Design review of the part built by this model. Coordinates are the model's own, in mm. A direction names the side the tool comes from. Give positions to 0.01 mm unless a question says otherwise; leave off trailing zeros. Order: outer loops, then holes, each group sorted by start corner. A loop starts at its lowest first (then second) coordinate and runs counter-clockwise, first axis right, second up. Notation, with made-up numbers: (11.5, -26) -> (43.5, -26) arc R35 cw to (43.5, 10) -> close; hole circle Ø4 at (33.5, 73.5). An arc over 180 degrees is marked (long way). Return JSON: item names as keys, results as strings.
```python
from build123d import *

# Parameters (mm, degrees)
F0_W     = 254
F0_H     = 100
F1_DEPTH = 25.4
F2_W     = 254
F2_H     = 100
F2_R     = 27.9579286296
F3_DEPTH = 25.4
F4_T     = -2.54


with BuildPart() as f1:
    # F0 (on Top) → F1 (new body)
    with BuildSketch(Plane.XY):
        with Locations((127, 50)):
            Rectangle(F0_W, F0_H)
    extrude(amount=F1_DEPTH)

    # F2 (on face) → F3 (intersect)
    with BuildSketch(Plane.XY.offset(25.4)):
        with Locations((127, 50)):
            Rectangle(F2_W, F2_H)
        with Locations((145.1960504055, 46.4161895216)):
            Circle(F2_R, mode=Mode.SUBTRACT)
    extrude(amount=-F3_DEPTH, mode=Mode.INTERSECT)

    # F4
    f4_openings = [f1.faces().sort_by_distance(p)[0] for p in [
        (2.729762, 50, 0),
    ]]
    offset(amount=F4_T, openings=f4_openings)


solid = f1.part
```
Item 1: Add section B-B (y = 57). Give the boundary of the cut face in (x, z).
Result set:
{"outline": "(0, 0) -> (2.54, 0) -> (2.54, 22.86) -> (116.59, 22.86) -> (116.59, 0) -> (119.32, 0) -> (119.32, 25.4) -> (0, 25.4) -> close; (171.07, 0) -> (173.8, 0) -> (173.8, 22.86) -> (251.46, 22.86) -> (251.46, 0) -> (254, 0) -> (254, 25.4) -> (171.07, 25.4) -> close"}
Item 2: Add section D-D (x = 68). Give the boundary of the cut face in (y, z).
Result set:
{"outline": "(0, 0) -> (2.54, 0) -> (2.54, 22.86) -> (97.46, 22.86) -> (97.46, 0) -> (100, 0) -> (100, 25.4) -> (0, 25.4) -> close"}
Item 3: Wall thickness on L1, parallel to Y at x = 195, z = 4.75; L2, parallel to Y at x = 167.5, z = 17.25; L3, parallel to Y at x = 169.5, z = 10: over which ranges is each line inside the solid? List them lowest first. Write a range as [from, to].
Result set:
{"L1": "y = [0, 2.54], [97.46, 100]", "L2": "y = [0, 2.54], [25.62, 29.56], [63.27, 67.22], [97.46, 100]", "L3": "y = [0, 2.54], [27.99, 32.6], [60.24, 64.84], [97.46, 100]"}
Item 4: Add section A-A (z = 17). Give the boundary of the cut face in (x, y).
Result set:
{"outline": "(0, 0) -> (254, 0) -> (254, 100) -> (0, 100) -> close; circle Ø61 at (145.2, 46.42); hole (2.54, 2.54) -> (251.46, 2.54) -> (251.46, 97.46) -> (2.54, 97.46) -> close; hole circle Ø55.92 at (145.2, 46.42)"}
Item 5: Machinability: for faces 1 (the face through (114.728, 47.757, 11.59)), 2 (the face through (0, 49, 13)), which of the approach directions +Z, -Z, +X, -X, +Y, -Y give a long, thin tool a straight path to every point of the face, cutting with its end or side? Answer none if there is none.
Result set:
{"face 1": "-Z", "face 2": "+Z, -Z, -X, +Y, -Y"}
Item 6: Add section C-C (x = 170.5). Give the boundary of the cut face in (y, z).
Result set:
{"outline": "(0, 0) -> (2.54, 0) -> (2.54, 22.86) -> (29.39, 22.86) -> (29.39, 0) -> (34.53, 0) -> (34.53, 25.4) -> (0, 25.4) -> close; (58.31, 0) -> (63.44, 0) -> (63.44, 22.86) -> (97.46, 22.86) -> (97.46, 0) -> (100, 0) -> (100, 25.4) -> (58.31, 25.4) -> close"}
Item 7: For pin 1 (7 mm diameter, centred on y = 31, z = 5.5, fed in from -X); pin 2 (8 mm diameter, centred on x = 204, y = 30, fed in from -Z), all flat-tipped, find the tip position at first contact; note any pin that passes through.
Result set:
{"pin 1": "stops at x = 0", "pin 2": "stops at z = 22.86"}
Item 8: Mouldability with a two-part tool opening along Y and no side actions: class faces 3 (the face through (125, 0, 13)), 4 (the face through (2.54, 49, 11)), 5 (the face through (125, 2.54, 11)), 6 (the face through (158.6, 21.7, 0)) as released by +Y, released by -Y, zero draft, split by the parting line, or undercut.
Result set:
{"face 3": "released by -Y", "face 4": "undercut", "face 5": "undercut", "face 6": "zero draft"}
